Drawing for the job (mm, zero at the part's lowest x, y, z). A direction names the side the tool comes from. Round coordinates to 2 decimals unless told otherwise and drop trailing zeros. Write each loop counter-clockwise with the first axis right and the second up, starting at its lowest first coordinate (ties: lowest second). Pieces come first, ordered by that corner, then holes. Notation, with made-up numbers: M -32.75,33 L 5.25,33 A27 ccw 5.25,63 Z; hole C 57,-38 d7. An arc over 180 degrees is marked long. Use a Markdown table: item, result. Add a question column.
1) Two-plate mould, pull along X, no slides. Class the marked faces 3, 4 and 5: released by +X, released by -X, zero draft, split by the parting line, or undercut.
2) Wall check: probe 1 along Z at (x, y) = (40, 13); probe 2 along Z at (x, y) = (60, 12); probe 3 along Z at (x, y) = (44, 17.5) (1 decimal). Give the ranges that are in metal, low to high.
3) Which spindle directions (+Z, -Z, +X, -X, +Y, -Y) get a long thin tool onto all of the face, cutting with end or side? Do the marked faces 1 and 2. Say none if no direction does.
4) Slice it at C-C on y = 7. Write the cut outline in (x, z), plus the area to 3 significant figures.
5) Drop flat-ended pins along their axis: P1, Ø8, axis at x = 51, z = 13.5, coming from the +Y side; P2, Ø12, axis at y = 13, z = 59.5, coming from the -X side; P3, Ø3, axis at x = 52.5, z = 12.5, coming from the +Y side; P4, Ø3.5, axis at x = 38, y = 17, coming from the -Z side. Give the stop position or say it passes through.
6) Slice it at B-B on y = 14.75. Write the cut outline in (x, z).
7) Slice it at A-A on x = 40. Write the cut outline in (y, z), plus the area to 3 significant figures.
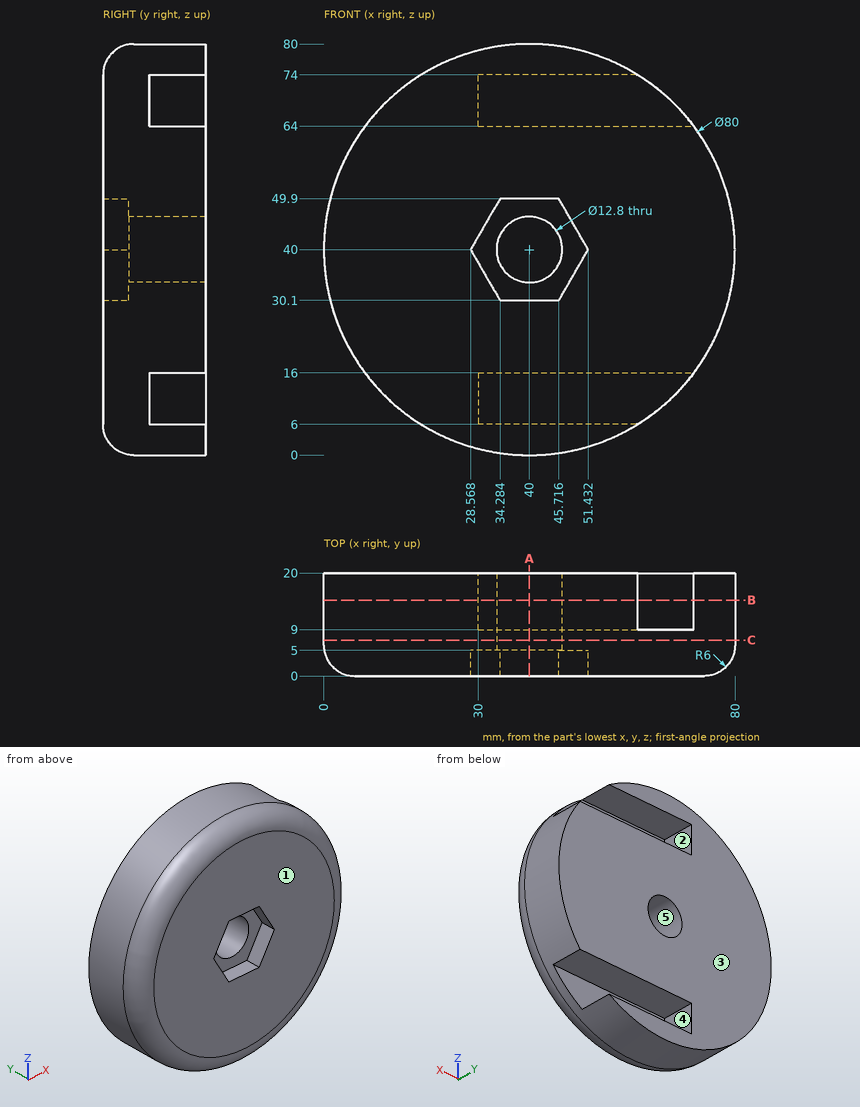
Entries:
| question | item | result |
|---|---|---|
| 1 | face 3 | zero draft |
| 1 | face 4 | released by +X |
| 1 | face 5 | undercut |
| 2 | probe 1 | z = 0 to 6, 16 to 33.6, 46.4 to 64, 74 to 80 |
| 2 | probe 2 | z = 5.36 to 6, 16 to 64, 74 to 74.64 |
| 2 | probe 3 | z = 0.2 to 6, 16 to 35, 45 to 64, 74 to 79.8 |
| 3 | face 1 | +Z, -Z, +X, -X, -Y |
| 3 | face 2 | +X, +Y |
| 4 | outline | C 40,40 d80; hole C 40,40 d12.8 |
| 4 | area | 4,900 mm^2 |
| 5 | P1 | stops at y = 20 |
| 5 | P2 | stops at x = 2.35 |
| 5 | P3 | stops at y = 9 |
| 5 | P4 | stops at z = 0 |
| 6 | outline | M 30,6 L 30,16 L 72,16 A40 ccw 72,64 L 30,64 L 30,74 L 61.07,74 A40 ccw long 61.07,6 Z; hole C 40,40 d12.8 |
| 7 | outline | M 0,6 A6 ccw 6,0 L 20,0 L 20,6 L 9,6 L 9,16 L 20,16 L 20,33.6 L 5,33.6 L 5,30.1 L 0,30.1 Z; M 0,49.9 L 5,49.9 L 5,46.4 L 20,46.4 L 20,64 L 9,64 L 9,74 L 20,74 L 20,80 L 6,80 A6 ccw 0,74 Z |
| 7 | area | 1,070 mm^2 |
